Geometry: see drawing. Coordinates: mm, zero at the bounding-box minimum. A direction names the side the tool comes from. Coordinates: 2 decimals unless noted, no trailing zeros. Order: outer loops, then holes, each group sorted by start corner. A loop starts at its lowest first (then second) coordinate and runs counter-clockwise, first axis right, second up. Notation, with made-up numbers: (11.5, 57) - (49.5, 57) arc R20 cw to (49.5, 93) - close; hole circle Ø6 at (56, 22.5). An arc over 180 degrees is marked (long way). Use a Markdown table: item, result. Add a question column.
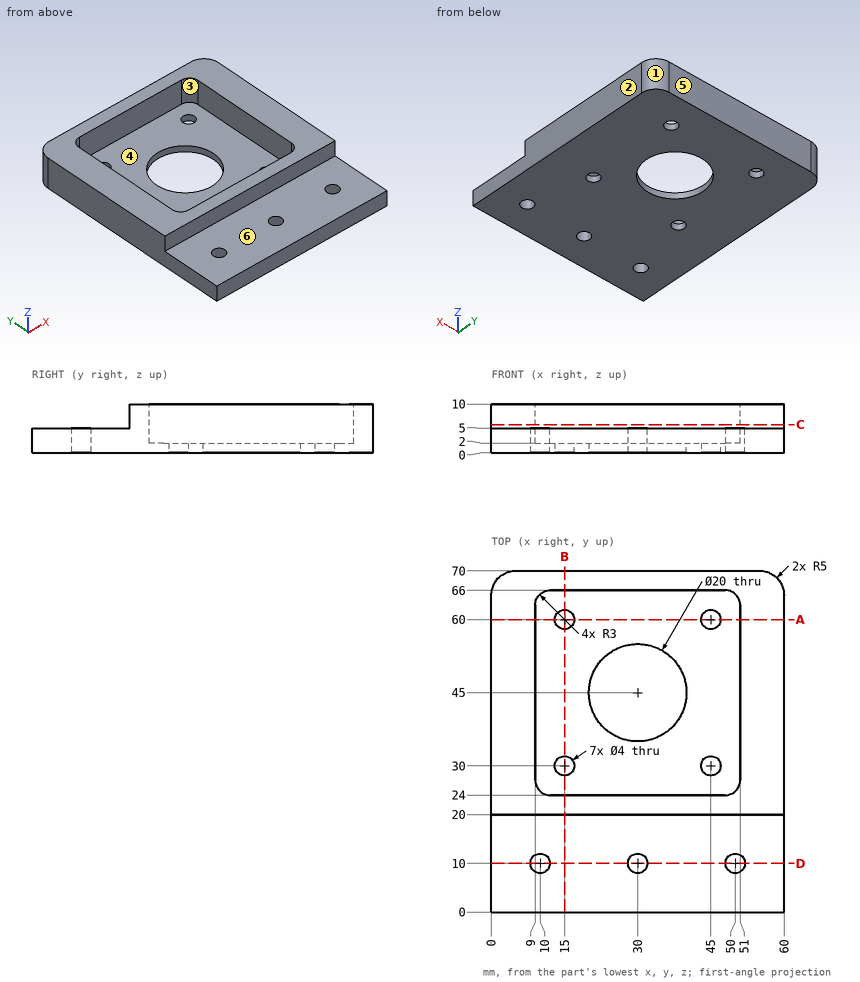
1) Contact query for flat-ended pins moving along their axis: P1, Ø12.5, axis at x = 21.5, y = 35.5, coming from the +Z side; P2, Ø5, axis at x = 42, z = 3, coming from the -Y side; P3, Ø3, axis at x = 45, y = 60, coming from the +Z side; P4, Ø10, axis at x = 17.5, y = 10.5, coming from the +Z side. Output: stop coordinate, or through.
2) Material intervals for L1, parallel to Y at x = 45, z = 1; L2, parallel to X at y = 30, z = 1.4; L3, parallel to Y at x = 30, z = 0.65, sorted ascending.
3) Cut plane A-A (y = 60). Return the cut outline in (x, z), and give its area (3 significant figures).
4) Cut plane B-B (x = 15). Return the cut outline in (y, z).
5) Cut plane C-C (z = 5.75). Return the cut outline in (x, y), and give its area (3 significant figures).
6) Pull-direction query (Y, two-part tool) for the marked faces 1, 2 and 3; classes: pulls with the +Y half, pulls with the -Y half, needs draft (parallel to the pull), parting line crosses it, or undercut.
7) Reachability of the marked faces 4, 5 and 6 from +Z, -Z, +X, -X, +Y, -Y: full face, straight path, thin tool, end or side. Return the list, or none.
8) Cut plane D-D (y = 10). Return the cut outline in (x, z), and give its area (3 significant figures).
Computed:
| question | item | result |
|---|---|---|
| 1 | P1 | stops at z = 2 |
| 1 | P2 | stops at y = 0 |
| 1 | P3 | passes through |
| 1 | P4 | stops at z = 5 |
| 2 | L1 | y = 0 to 28, 32 to 58, 62 to 70 |
| 2 | L2 | x = 0 to 13, 17 to 43, 47 to 60 |
| 2 | L3 | y = 0 to 8, 12 to 35, 55 to 70 |
| 3 | outline | (0, 0) - (13, 0) - (13, 2) - (9, 2) - (9, 10) - (0, 10) - close; (17, 0) - (43, 0) - (43, 2) - (17, 2) - close; (47, 0) - (60, 0) - (60, 10) - (51, 10) - (51, 2) - (47, 2) - close |
| 3 | area | 248 mm2 |
| 4 | outline | (0, 0) - (28, 0) - (28, 2) - (24, 2) - (24, 10) - (20, 10) - (20, 5) - (0, 5) - close; (32, 0) - (58, 0) - (58, 2) - (32, 2) - close; (62, 0) - (70, 0) - (70, 10) - (66, 10) - (66, 2) - (62, 2) - close |
| 5 | outline | (0, 20) - (60, 20) - (60, 65) arc R5 ccw to (55, 70) - (5, 70) arc R5 ccw to (0, 65) - close; hole (9, 27) arc R3 ccw to (12, 24) - (48, 24) arc R3 ccw to (51, 27) - (51, 63) arc R3 ccw to (48, 66) - (12, 66) arc R3 ccw to (9, 63) - close |
| 5 | area | 1,230 mm2 |
| 6 | face 1 | pulls with the +Y half |
| 6 | face 2 | needs draft |
| 6 | face 3 | undercut |
| 7 | face 4 | +Z |
| 7 | face 5 | +Z, -Z, +X, -X, +Y |
| 7 | face 6 | +Z, +X, -X, -Y |
| 8 | outline | (0, 0) - (8, 0) - (8, 5) - (0, 5) - close; (12, 0) - (28, 0) - (28, 5) - (12, 5) - close; (32, 0) - (48, 0) - (48, 5) - (32, 5) - close; (52, 0) - (60, 0) - (60, 5) - (52, 5) - close |
| 8 | area | 240 mm2 |
